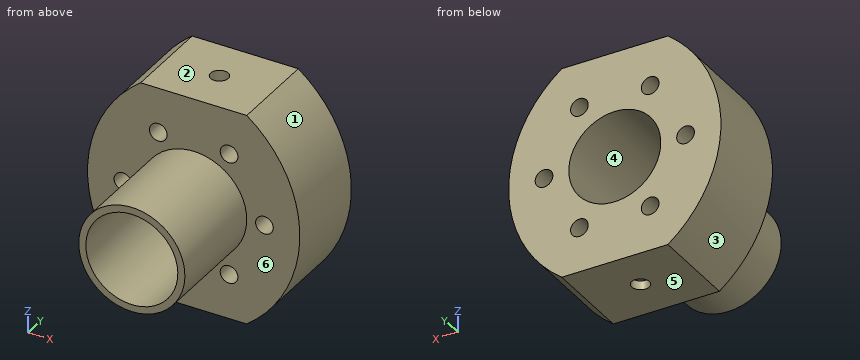
from build123d import *

# Parameters (mm, degrees)
SALIENTE_EXTRUIR2_DEPTH = 12.5
CROQUIS31_R             = 15
SALIENTE_EXTRUIR3_DEPTH = 30
CROQUIS8_R              = 13
CORTAR_EXTRUIR2_DEPTH   = 100
CROQUIS33_R             = 2.5
CORTAR_EXTRUIR9_DEPTH   = 2.5
CORTAR_EXTRUIR10_START  = -5
CROQUIS34_R             = 2.5
CORTAR_EXTRUIR10_DEPTH  = 5
CROQUIS35_R             = 2.5
CORTAR_EXTRUIR11_DEPTH  = 25


with BuildPart() as part:
    # Croquis1 → Saliente-Extruir2 (new, symmetric)
    with BuildSketch(Plane(origin=(0, 0, 0), x_dir=(1, 0, 0), z_dir=(0, 1, 0))):
        with BuildLine():
            Line((-15, -30), (15, -30))
            ThreePointArc((15, -30), (30, 0), (15, 30))
            Line((15, 30), (-15, 30))
            ThreePointArc((-15, 30), (-30, 0), (-15, -30))
        make_face()
    extrude(amount=SALIENTE_EXTRUIR2_DEPTH, both=True)

    # Croquis31 → Saliente-Extruir3 (add)
    with BuildSketch(Plane(origin=(0, -12.5, 0), x_dir=(-1, 0, 0), z_dir=(0, -1, 0))):
        with Locations(Location((0, 0, 0), (0, 0, 90))):
            Circle(CROQUIS31_R)
    extrude(amount=SALIENTE_EXTRUIR3_DEPTH)

    # Croquis8 → Cortar-Extruir2 (cut)
    with BuildSketch(Plane(origin=(0, 12.5, 0), x_dir=(1, 0, 0), z_dir=(0, 1, 0))):
        with Locations(Location((0, 0, 0), (0, 0, 270))):
            Circle(CROQUIS8_R)
    extrude(amount=-CORTAR_EXTRUIR2_DEPTH, mode=Mode.SUBTRACT)

    # Croquis33 → Cortar-Extruir9 (cut, symmetric)
    with BuildSketch(Plane(origin=(0, 0, -30), x_dir=(-1, 0, 0), z_dir=(0, 0, -1))):
        Circle(CROQUIS33_R)
    extrude(amount=CORTAR_EXTRUIR9_DEPTH, both=True, mode=Mode.SUBTRACT)

    # Croquis34 → Cortar-Extruir10 (cut)
    with BuildSketch(Plane.XY.offset(30).offset(CORTAR_EXTRUIR10_START)):
        with Locations(Location((0, 0, 0), (0, 0, 180))):
            Circle(CROQUIS34_R)
    extrude(amount=CORTAR_EXTRUIR10_DEPTH, mode=Mode.SUBTRACT)

    # Croquis35 → Cortar-Extruir11 (cut)
    with BuildSketch(Plane(origin=(0, 12.5, 0), x_dir=(1, 0, 0), z_dir=(0, 1, 0))):
        with Locations(Location((20, 0, 0), (0, 0, 270))):
            Circle(CROQUIS35_R)
        with Locations(Location((-20, 0, 0), (0, 0, 270))):
            Circle(CROQUIS35_R)
        with Locations(Location((-10, 17.320508076, 0), (0, 0, 270))):
            Circle(CROQUIS35_R)
        with Locations(Location((10, 17.320508076, 0), (0, 0, 270))):
            Circle(CROQUIS35_R)
        with Locations(Location((10, -17.320508076, 0), (0, 0, 270))):
            Circle(CROQUIS35_R)
        with Locations(Location((-10, -17.320508076, 0), (0, 0, 270))):
            Circle(CROQUIS35_R)
    extrude(amount=-CORTAR_EXTRUIR11_DEPTH, mode=Mode.SUBTRACT)


solid = part.part
Source: CAD feature listing. Evaluate the final solid. Frame: model axes, mm. Face numbers are marked on the shaded views. A direction names the side the tool comes from. Round coordinates to 2 decimals unless told otherwise and drop trailing zeros. Loops run counter-clockwise (first coordinate to the right, second up) from the corner with the lowest first, then second, coordinate; pieces in that order, holes last. Notation, with made-up numbers: M 35,57.25 L 68,57.25 A22 cw 68,73.25 Z; hole C 47,25.25 d4. An arc over 180 degrees is marked long. Return JSON: item names as keys, results as strings. Group by question number.
1. Section query B-B on z = 0. Output: boundary loops of the cut face in (x, y).
2. Material intervals for line 1 along Y through (x, z) = (0, 27); line 2 along Y through (x, z) = (-22, 16); line 3 along X through (y, z) = (8, -19.5), sorted ascending. Write a range as from..to.
3. Section query D-D on y = -34. Output: boundary loops of the cut face in (x, z), and give its area (3 significant figures).
4. Section query C-C on y = 3.5. Output: boundary loops of the cut face in (x, z), and give its area (3 significant figures).
5. Section query A-A on x = 0. Output: boundary loops of the cut face in (y, z), and give its area (4 significant figures).
6. Pin query (flat end, axial travel): pin 1 (2.5 mm diameter, centred on x = 1, y = -1, fed in from +Z); pin 2 (6.5 mm diameter, centred on x = -10, z = 17.32, fed in from -Y); pin 3 (4.5 mm diameter, centred on x = 0, y = 0, fed in from -Z); pin 4 (4.5 mm diameter, centred on x = 0, y = 0, fed in from +Z). Return the tip coordinate at first contact, or that it passes through.
7. Mould query, pull axis X, two halves, no side actions, for the marked faces 1, 2, 3 and 4. Classes: released by +X, released by -X, zero draft, split by the parting line, or undercut.
8. Reachability of the marked faces 5 and 6 from +Z, -Z, +X, -X, +Y, -Y: full face, straight path, thin tool, end or side. Return the list, or none.
Checks:
{
 "1": {"outline": "M -30,-12.5 L -22.5,-12.5 L -22.5,12.5 L -30,12.5 Z; M -17.5,-12.5 L -15,-12.5 L -15,-42.5 L -13,-42.5 L -13,12.5 L -17.5,12.5 Z; M 13,-42.5 L 15,-42.5 L 15,-12.5 L 17.5,-12.5 L 17.5,12.5 L 13,12.5 Z; M 22.5,-12.5 L 30,-12.5 L 30,12.5 L 22.5,12.5 Z"},
 "2": {"line 1": "y = -12.5..-2.5, 2.5..12.5", "line 2": "y = -12.5..12.5", "line 3": "x = -24.53..-11.22, -8.78..8.78, 11.22..24.53"},
 "3": {"outline": "C 0,0 d30; hole C 0,0 d26", "area": "176 mm²"},
 "4": {"outline": "M -15,-30 L 15,-30 A37.5 ccw 15,30 L -15,30 A37.5 ccw Z; hole C -20,0 d5; hole C 0,0 d26; hole C -10,-17.32 d5; hole C -10,17.32 d5; hole C 10,-17.32 d5; hole C 10,17.32 d5; hole C 20,0 d5", "area": "2,410 mm²"},
 "5": {"outline": "M -42.5,-15 L -12.5,-15 L -12.5,-30 L -2.5,-30 L -2.5,-27.5 L 2.5,-27.5 L 2.5,-30 L 12.5,-30 L 12.5,-13 L -42.5,-13 Z; M -42.5,13 L 12.5,13 L 12.5,30 L 2.5,30 L 2.5,25 L -2.5,25 L -2.5,30 L -12.5,30 L -12.5,15 L -42.5,15 Z", "area": "932.5 mm²"},
 "6": {"pin 1": "stops at z = 30", "pin 2": "stops at y = -12.5", "pin 3": "stops at z = -27.5", "pin 4": "stops at z = 25"},
 "7": {"face 1": "released by +X", "face 2": "zero draft", "face 3": "released by -X", "face 4": "undercut"},
 "8": {"face 5": "-Z, +X, -X, +Y, -Y", "face 6": "-Y"}
}
